Geometry check sheet. Reference: the model listing, model coordinates, mm. A direction names the side the tool comes from. Give positions to 0.01 mm unless a question says otherwise; leave off trailing zeros. Order: outer loops, then holes, each group sorted by start corner. A loop starts at its lowest first (then second) coordinate and runs counter-clockwise, first axis right, second up. Notation, with made-up numbers: M 1,86.25 L 31,86.25 A19 cw 31,105.25 Z; hole C 11.25,-22.5 d2. An arc over 180 degrees is marked long. Answer as CSV lines item,"result". Start each with the question number.
Q1. Section check C-C, the plane z = 13. Record the boundary of the cut face in (x, y), then the cut area to 3 significant figures.
Q2. Thickness scan on line 1 (X direction, y = 35, z = 1); line 2 (Y direction, x = -616, z = 20.25). Record the ranges inside material, lowest first.
Q3. Go/stop test with flat-tipped pins: pin 1 (1.5 mm diameter, centred on x = -1, z = 1.5, fed in from +Y); pin 2 (12 mm diameter, centred on x = 46, z = 17.5, fed in from +Y); pin 3 (2 mm diameter, centred on x = -352.5, y = 59.5, fed in from +Z). Record where each tip stops, or that it passes through.
Q4. Section check B-B, the plane x = 175. Record the boundary of the cut face in (y, z).
Q5. Set-up check for faces 1 (the flat face through (-10, 37, 3)), 2 (the flat face through (10, 0, 18)): record each of +Z, -Z, +X, -X, +Y, -Y from which the full face is reachable in a straight line by a thin tool's end or side.
Q6. Section check A-A, the plane y = 42. Record the boundary of the cut face in (x, z), then the cut area to 3 significant figures.
Autodesk Inventor part; units mm, degrees
ref_plane "YZ Plane" through (0, 0, 0) normal (1, 0, 0) x (0, 1, 0)
ref_plane "XZ Plane" through (0, 0, 0) normal (0, 1, 0) x (-1, 0, 0)
ref_plane "XY Plane" through (0, 0, 0) normal (0, 0, 1) x (1, 0, 0)
sketch "Sketch1" plane through (0, 0, 0) normal (0, 0, 1) x (1, 0, 0)
  line L0 (-750, 67.3571) -> (750, 67.3571)
  line L1 (750, 67.3571) -> (750, 0)
  line L2 (750, 0) -> (-750, 0)
  line L3 (-750, 0) -> (-750, 67.3571)
  point P0 (0, 0)
  point P1 (0, 0)
  dimension "d0" = 1500
  dimension "d1" = 67.3571
extrude "Plate1" add sketch "Sketch1" along normal blind 3
sketch "Sketch2" plane through (750, 3, 0) normal (0, -1, 0) x (1, 0, 0)
  line L0 (-1500, 0) -> (0, 0)
  line L1 (0, 0) -> (0, 30)
  line L2 (0, 30) -> (-1500, 30)
  line L3 (-1500, 30) -> (-1500, 0)
edge flange "Flange1" height 30 angle 90 thickness 3 bend radius 3 thickness toward (0, -1, 0) relief tear relief width 3 relief depth 1.5 edges at (0, 0, 3) wall of the first edge with corners at (-750, 3, 0) (750, 3, 0) (750, 3, 30) (-750, 3, 30)
bend "Bend1"
corner "Corner1"
sketch "Sketch5" plane through (0, 0, 0) normal (0, 0, -1) x (-1, 0, 0)
  line L0 (750, 67.3571) -> (-750, 67.3571)
  line L1 (500, 67.3571) -> (500, 31)
  line L2 (500, 31) -> (503, 31)
  line L3 (503, 31) -> (503, 67.3571)
  line L4 (750, 0) -> (-750, 0)
  point P0 (0, 0)
  dimension "d18" = 3
  dimension "d19" = 247
  dimension "d20" = 31
extrude "Extrusion1" cut sketch "Sketch5" against normal through all
pattern_linear "Rectangular Pattern1" count 3 spacing 500 along (1, 0, 0) of "Extrusion1"
sketch "Sketch6" plane through (0, 0, 0) normal (0, 0, -1) x (-1, 0, 0)
  line L0 (-750, 67.3571) -> (-750, 6)
  circle A0 centre (-750, 67.3571) radius 15
  line L1 (-750, 67.3571) -> (750, 67.3571)
  point P0 (0, 0)
  point P1 (-500, 67.3571)
  point P2 (-735, 67.3571)
  point P3 (-750, 52.3571)
  dimension "d24" = 30
extrude "Extrusion2" cut sketch "Sketch6" against normal through all contours L1 A0 L0 picked at (-740.1254, 66.2445)
mirror "Mirror1" about plane through (0, 0, 0) normal (1, 0, 0) of "Extrusion2"
equation "\"d1\" = Стрингер_3"
equation "\"d18\" = Thickness"
equation "\"d2\" = Thickness"
equation "\"d3\" = BendReliefWidth"
equation "\"d4\" = BendReliefDepth"
equation "\"d5\" = MinimumRemnant"
equation "\"d6\" = TransitionRadius"
equation "\"d9\" = BendRadius"
equation "\"d10\" = CornerReliefSize"
equation "\"d11\" = GapSize"
equation "\"d12\" = JacobiRadiusSize"
equation "\"BendRadius\" = Thickness"
equation "\"BendReliefWidth\" = Thickness"
equation "\"BendReliefDepth\" = 0.5 * Thickness"
equation "\"CornerReliefSize\" = 4 * Thickness"
equation "\"MinimumRemnant\" = 2 * Thickness"
equation "\"TransitionRadius\" = BendRadius"
equation "\"JacobiRadiusSize\" = BendRadius"
equation "\"GapSize\" = Thickness"
properties part number "МОО 053 стрингер борт 31"
Answer block:
1,outline,"M -750,0 L 750,0 L 750,3 L -750,3 Z"
1,area,"4,500 mm2"
2,line 1,"x = -750 to -503, -500 to -3, 0 to 497, 500 to 750"
2,line 2,"y = 0 to 3"
3,pin 1,"stops at y = 31"
3,pin 2,"stops at y = 3"
3,pin 3,"stops at z = 3"
4,outline,"M 0,6 A6 ccw 6,0 L 67.36,0 L 67.36,3 L 6,3 A3 cw 3,6 L 3,30 L 0,30 Z"
5,face 1,"+Z, +X, -X, +Y"
5,face 2,"+Z, -Z, +X, -X, -Y"
6,outline,"M -750,0 L -503,0 L -503,3 L -750,3 Z; M -500,0 L -3,0 L -3,3 L -500,3 Z; M 0,0 L 497,0 L 497,3 L 0,3 Z; M 500,0 L 750,0 L 750,3 L 500,3 Z"
6,area,"4,470 mm2"
